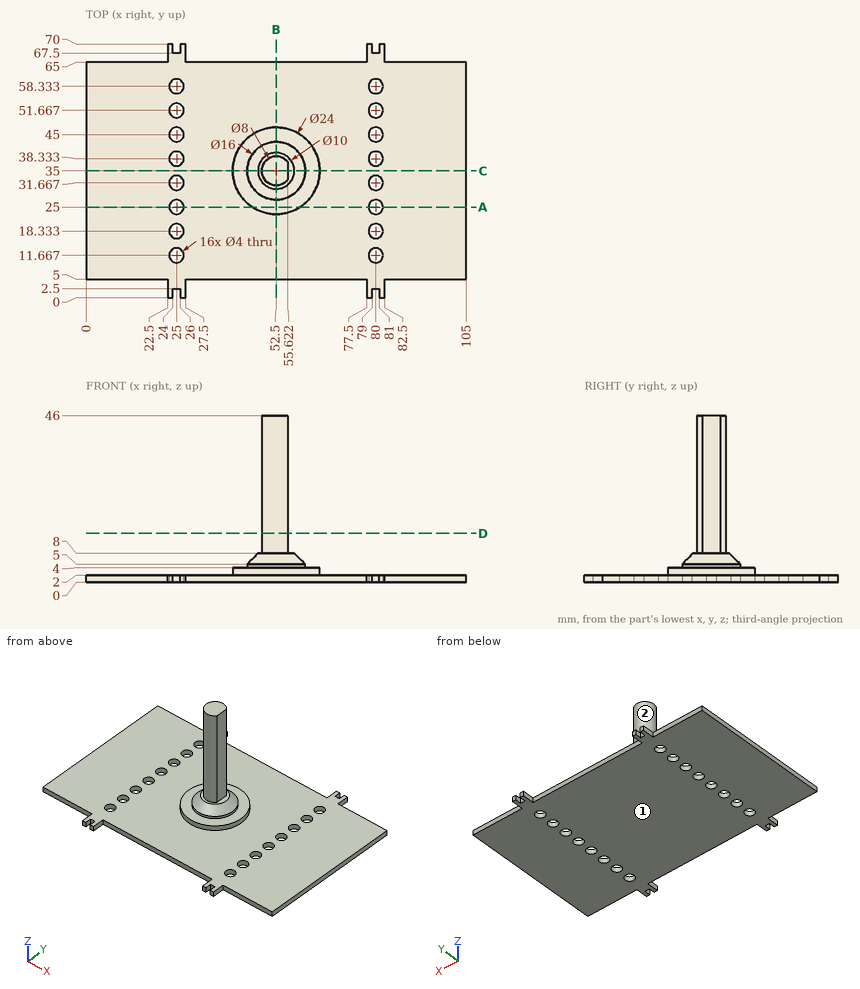
Print and shaded views of the part. All mm, measured from the part's lowest x, y and z. A direction names the side the tool comes from. Coordinates: 2 decimals unless noted, no trailing zeros. Loops run counter-clockwise (first coordinate to the right, second up) from the corner with the lowest first, then second, coordinate; pieces in that order, holes last. Notation, with made-up numbers: M -0.5,80 L 20.5,80 A23 ccw 20.5,91 Z; hole C 33,31.5 d2. An arc over 180 degrees is marked long. Use a Markdown table: item, result. Add a question column.
Q1. Cut at D-D (z = 13.5). Write the cut outline in (x, y).
Q2. Which spindle directions (+Z, -Z, +X, -X, +Y, -Y) get a long thin tool onto all of the face, cutting with end or side? Do the marked faces 1 and 2. Say none if no direction does.
Q3. Probe L1, parallel to Z at x = 96, y = 27; L2, parallel to X at y = 35.5, z = 39. List the from-to ranges inside material, lowest first.
Q4. Pin check, flat tips, straight feed: P1, Ø6.5, axis at x = 25, y = 45, coming from the +Z side; P2, Ø6.5, axis at x = 80, y = 25, coming from the -Z side; P3, Ø0.6, axis at y = 1, z = 1, coming from the -X side; P4, Ø0.6, axis at x = 25, z = 1, coming from the -Y side. Stop position of each tip, or through.
Q5. Cut at C-C (y = 35). Write the cut outline in (x, z).
Q6. Cut at A-A (y = 25). Write the cut outline in (x, z).
Q7. Cut at B-B (x = 52.5). Write the cut outline in (y, z), and give its area (3 significant figures).
Worked out:
| question | item | result |
|---|---|---|
| 1 | outline | M 55.62,32.5 L 55.62,37.5 A4 ccw long Z |
| 2 | face 1 | -Z, +X, -X, +Y, -Y |
| 2 | face 2 | +Z |
| 3 | L1 | z = 0 to 2 |
| 3 | L2 | x = 48.53 to 55.62 |
| 4 | P1 | stops at z = 2 |
| 4 | P2 | stops at z = 0 |
| 4 | P3 | stops at x = 22.5 |
| 4 | P4 | stops at y = 2.5 |
| 5 | outline | M 0,0 L 105,0 L 105,2 L 64.5,2 L 64.5,4 L 60.5,4 L 60.5,5 L 57.5,8 L 55.62,8 L 55.62,46 L 48.5,46 L 48.5,8 L 47.5,8 L 44.5,5 L 44.5,4 L 40.5,4 L 40.5,2 L 0,2 Z |
| 6 | outline | M 0,0 L 23,0 L 23,2 L 0,2 Z; M 27,0 L 78,0 L 78,2 L 59.13,2 L 59.13,4 L 45.87,4 L 45.87,2 L 27,2 Z; M 82,0 L 105,0 L 105,2 L 82,2 Z |
| 7 | outline | M 5,0 L 65,0 L 65,2 L 47,2 L 47,4 L 43,4 L 43,5 L 40,8 L 39,8 L 39,46 L 31,46 L 31,8 L 30,8 L 27,5 L 27,4 L 23,4 L 23,2 L 5,2 Z |
| 7 | area | 527 mm2 |
